Part model, mm, in its own coordinate system. Face numbers are marked on the shaded views. A direction names the side the tool comes from. Round coordinates to 2 decimals unless told otherwise and drop trailing zeros. Write each loop counter-clockwise with the first axis right and the second up, starting at its lowest first coordinate (ties: lowest second). Pieces come first, ordered by that corner, then holes. Notation, with made-up numbers: (-16.5, -8.75) -> (-7.5, -8.75) arc R35 ccw to (-7.5, 28.25) -> close; hole circle Ø7 at (-5, -24.75). An arc over 180 degrees is marked (long way). Use CSV: the item, a comma, the result in double quotes. Start each with the question number.
(1) Saw through at B-B (x = 66). Give the cut face in (y, z).
(2) Saw through at A-A (x = -43). Give the cut face in (y, z), plus the area to 3 significant figures.
(3) Which spindle directions (+Z, -Z, +X, -X, +Y, -Y) get a long thin tool onto all of the face, cutting with end or side? Do the marked faces 4, 5 and 6. Say none if no direction does.
(4) Saw through at C-C (x = 0.5). Give the cut face in (y, z), plus the area to 3 significant figures.
(5) Two-plate mould, pull along X, no slides. Class the marked faces 1, 2 and 3: released by +X, released by -X, zero draft, split by the parting line, or undercut.
(6) Probe line 1 (Z direction, x = -48.25, y = 0); line 2 (X direction, y = -8.5, z = -8.5); line 3 (X direction, y = -0.5, z = -10.5). List the from-to ranges inside material, lowest first. Write a range as [from, to].
(7) Drop flat-ended pins along their axis: pin 1 (3 mm diameter, centred on y = 1.5, z = -20.5, fed in from +X); pin 2 (1 mm diameter, centred on y = 15, z = 0, fed in from +X); pin 3 (2.5 mm diameter, centred on x = -29, z = 2, fed in from +Y). Give the stop position or say it passes through.
```python
from build123d import *

# Parameters (mm, degrees)
F0_W     = 20
F0_H     = 11.0503323376
F0_H_2   = 1.4496676624
F0_W_2   = 35
F0_H_3   = 23.5
F0_W_3   = 10
F0_H_4   = 14
F2_DEPTH = 5
F3_DEPTH = 5
F4_DEPTH = 10
F6_R     = 1.27
F7_R     = 11.2300002947
F8_DEPTH = 15.24
F5_R     = 2.9447713958
F9_DEPTH = 1.778
F10_R    = 0.5518892204


with BuildPart() as f1:
    # F0 (on Top) → F1 (revolve)
    with BuildSketch(Plane.XY):
        with Locations((-45.1154029071, 5.5251661688)):
            Rectangle(F0_W, F0_H)
        with Locations((-45.1154029071, 11.7751661688)):
            Rectangle(F0_W, F0_H_2)
        Polygon((-35.1154029071, 11.0503323376), (-35.1154029071, 0), (-28.1154029071, 0), (-28.1154029071, 11.0503323376), (-34.2071130872, 11.0503323376), align=None)
        Polygon((-28.1154029071, 11.0503323376), (-28.1154029071, 0), (-17.1154029071, 0), (6.8845970929, 0), (6.8845970929, 23.5), (-17.1154029071, 14.9630850315), align=None)
        with Locations((24.3845970929, 11.75)):
            Rectangle(F0_W_2, F0_H_3)
        Polygon((41.8845970929, 23.5), (41.8845970929, 0), (51.8845970929, 0), (51.8845970929, 26), align=None)
        Polygon((51.8845970929, 26), (51.8845970929, 0), (106.8845970929, 0), (113.8845970929, 0), (113.8845970929, 14), (106.8845970929, 26), align=None)
        with Locations((118.8845970929, 7)):
            Rectangle(F0_W_3, F0_H_4)
    revolve(axis=Axis((34.3845970929, 0, 0), (1, 0, 0)))



with BuildPart() as f2:
    # F0 (on Top) → F2 (new body)
    with BuildSketch(Plane.XY):
        Polygon((-34.2071130872, 11.0503323376), (-28.1154029071, 11.0503323376), (-17.1154029071, 14.9630850315), (-26.2071130872, 18.0503323376), (-34.2071130872, 18.0503323376), align=None)
    extrude(amount=F2_DEPTH)


with BuildPart() as f1_1:
    add(f1.part)

    add(f2.part)  # F3 merges F2
    # F0 (on Top) → F3 (join)
    with BuildSketch(Plane.XY):
        Polygon((-34.2071130872, 11.0503323376), (-28.1154029071, 11.0503323376), (-17.1154029071, 14.9630850315), (-26.2071130872, 18.0503323376), (-34.2071130872, 18.0503323376), align=None)
    extrude(amount=-F3_DEPTH)

    # F4 (add): faces of the model
    f4_faces = [f1_1.faces().sort_by_distance(p)[0] for p in [
        (-31.1612579972, 11.0503323376, 2.5),
        (-31.1612579972, 11.0503323376, -2.5),
        (-22.6154029071, 13.0067086846, 2.5),
        (-22.6154029071, 13.0067086846, -2.5),
    ]]
    extrude(f4_faces, amount=F4_DEPTH, dir=(0, -1, 0))

    # F6
    f6_edges = [f1_1.edges().sort_by_distance(p)[0] for p in [
        (-34.207113, 13.952383, 5),
        (-34.207113, 13.952383, -5),
        (-34.661258, 11.050332, 0),
        (123.884597, -14, 0),
        (106.884597, -26, 0),
        (51.884597, -26, 0),
        (6.884597, -23.5, 0),
    ]]
    fillet(f6_edges, radius=F6_R)

    # F7 (on face) → F8 (cut)
    with BuildSketch(Plane(origin=(-55.1154029071, 0, 0), x_dir=(0, -1, 0), z_dir=(-1, 0, 0))):
        Circle(F7_R)
    extrude(amount=-F8_DEPTH, mode=Mode.SUBTRACT)

    # F5 (on face) → F9 (join)
    with BuildSketch(Plane(origin=(0, 18.0503323376, 0), x_dir=(-1, 0, 0), z_dir=(0, 1, 0))):
        with Locations((30.1491450518, 0)):
            Circle(F5_R)
    extrude(amount=F9_DEPTH)

    # F10
    f10_edges = [f1_1.edges().sort_by_distance(p)[0] for p in [
        (-27.204374, 19.828332, 0),
    ]]
    fillet(f10_edges, radius=F10_R)


solid = f1_1.part
```
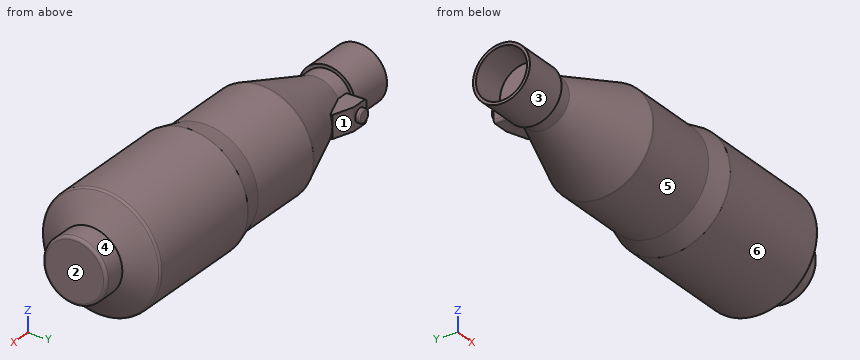
Answers:
1,outline,"circle Ø52 at (0, 0)"
2,outline,"circle Ø25 at (0, 0); hole circle Ø22.46 at (0, 0)"
2,area,"94.7 mm²"
3,face 4,"+X"
3,face 5,"-X"
3,face 6,"+X, -X"
4,outline,"circle Ø42.46 at (0, 0)"
4,area,"1,420 mm²"
5,face 1,"undercut"
5,face 2,"released by +X"
5,face 3,"zero draft"
6,line 1,"z = [-12.5, -11.23], [11.23, 12.5]"
6,line 2,"x = [-55.12, -35.12], [-25.39, 123.88]"
6,line 3,"x = [-39.88, 123.88]"
7,pin 1,"stops at x = 110.94"
7,pin 2,"stops at x = 113.59"
7,pin 3,"stops at y = 19.83"
